Geometry: final body of the model. Coordinates: model frame, mm. A direction names the side the tool comes from. Coordinates: 2 decimals unless noted, no trailing zeros. Order: outer loops, then holes, each group sorted by start corner. A loop starts at its lowest first (then second) coordinate and runs counter-clockwise, first axis right, second up. Notation, with made-up numbers: (87, 77) - (141, 77) arc R27 cw to (141, 108) - close; hole circle Ø10 at (84, 36.25). An arc over 180 degrees is marked (long way). Use a Markdown table: item, result. Add a question column.
```python
from build123d import *

# Parameters (mm, degrees)
SKETCH1_R           = 9
SKETCH1_R_2         = 2
SKETCH1_R_3         = 2.25
BOSS_EXTRUDE1_DEPTH = 2.5
SKETCH2_R           = 9
BOSS_EXTRUDE2_DEPTH = 3
SKETCH3_R           = 1
CUT_EXTRUDE1_DEPTH  = 6.5


with BuildPart() as part:
    # Sketch1 → Boss-Extrude1 (new body)
    with BuildSketch(Plane(origin=(0, 0, 0), x_dir=(1, 0, 0), z_dir=(0, 1, 0))):
        Circle(SKETCH1_R)
        with Locations((-4.763139721, -2.75)):
            Circle(SKETCH1_R_2, mode=Mode.SUBTRACT)
        with Locations((0, 5.5)):
            Circle(SKETCH1_R_2, mode=Mode.SUBTRACT)
        with Locations((4.763139721, -2.75)):
            Circle(SKETCH1_R_2, mode=Mode.SUBTRACT)
        Circle(SKETCH1_R_3, mode=Mode.SUBTRACT)
    extrude(amount=BOSS_EXTRUDE1_DEPTH)

    # Sketch2 → Boss-Extrude2 (add)
    with BuildSketch(Plane(origin=(0, 2.5, 0), x_dir=(1, 0, 0), z_dir=(0, 1, 0))):
        Circle(SKETCH2_R)
    extrude(amount=BOSS_EXTRUDE2_DEPTH)

    # Sketch3 → Cut-Extrude1 (cut, through all)
    with BuildSketch(Plane(origin=(0, 5.5, 0), x_dir=(1, 0, 0), z_dir=(0, 1, 0))):
        Circle(SKETCH3_R)
    extrude(amount=-CUT_EXTRUDE1_DEPTH, mode=Mode.SUBTRACT)


solid = part.part
```
1) First-contact query: pin 1 (1.5 mm diameter, centred on x = -3.5, y = 4, fed in from -Z); pin 2 (1 mm diameter, centred on x = 2.5, y = 4, fed in from -Z); pin 3 (2.5 mm diameter, centred on x = 0, z = 0, fed in from -Y); pin 4 (1.6 mm diameter, centred on x = 0, z = 0, fed in from +Y). Flat tips, straight axial feed; report the tip coordinate or a pass-through.
2) Section query B-B (x = 0). Return the cut outline in (y, z).
3) Access query for faces 1 (the flat face through (0, 5.5, 2)), 2 (the cylindrical face through (-0.26, 1.232, -7.483)). Directions: +Z, -Z, +X, -X, +Y, -Y. A direction counts if a zero-diameter tool reaches every point of the face in a straight line with its end or side. Return the directions, or none.
4) Section query A-A (z = 0). Return the cut outline in (x, y).
5) Draft query along X for faces 3 (the flat face through (-1, 2.5, 1)), 4 (the cylindrical face through (-1.172, 2.712, -8.923)), 5 (the flat face through (2, 0, 2)). Return one class per face: released by +X, released by -X, zero draft, split by the parting line, or undercut.
6) Section query D-D (y = 4.6). Return the cut outline in (x, z), and give its area (3 significant figures).
7) Line query: line 1 (Z direction, x = 0, y = 2.05); line 2 (X direction, y = 0.6, z = 0); line 3 (Z direction, x = -0.5, y = 0.7). Output: solid intervals per line, ascending. Write a range as from..to.
8) Section query C-C (y = 0.5). Return the cut outline in (x, z), and give its area (3 significant figures).
From the geometry:
| question | item | result |
|---|---|---|
| 1 | pin 1 | stops at z = -8.57 |
| 1 | pin 2 | stops at z = -8.77 |
| 1 | pin 3 | stops at y = 2.5 |
| 1 | pin 4 | passes through |
| 2 | outline | (0, -9) - (5.5, -9) - (5.5, -1) - (2.5, -1) - (2.5, -2.25) - (0, -2.25) - (0, -3.5) - (2.5, -3.5) - (2.5, -7.5) - (0, -7.5) - close; (0, 2.25) - (2.5, 2.25) - (2.5, 1) - (5.5, 1) - (5.5, 9) - (0, 9) - close |
| 3 | face 1 | +Z, -Z, +X, -X, +Y |
| 3 | face 2 | -Y |
| 4 | outline | (-9, 0) - (-2.25, 0) - (-2.25, 2.5) - (-1, 2.5) - (-1, 5.5) - (-9, 5.5) - close; (1, 2.5) - (2.25, 2.5) - (2.25, 0) - (9, 0) - (9, 5.5) - (1, 5.5) - close |
| 5 | face 3 | undercut |
| 5 | face 4 | split by the parting line |
| 5 | face 5 | zero draft |
| 6 | outline | circle Ø18 at (0, 0); hole circle Ø2 at (0, 0) |
| 6 | area | 251 mm^2 |
| 7 | line 1 | z = -9..-7.5, -3.5..-2.25, 2.25..9 |
| 7 | line 2 | x = -9..-2.25, 2.25..9 |
| 7 | line 3 | z = -8.99..-7.44, -3.56..-2.19, 2.19..8.99 |
| 8 | outline | circle Ø18 at (0, 0); hole circle Ø4 at (-4.76, 2.75); hole circle Ø4.5 at (0, 0); hole circle Ø4 at (0, -5.5); hole circle Ø4 at (4.76, 2.75) |
| 8 | area | 201 mm^2 |
